The listing builds one solid part. Answer for the finished solid, in the listing's coordinates (mm). Face numbers are marked on the shaded views. Give positions to 0.01 mm unless a question says otherwise; leave off trailing zeros. Loops run counter-clockwise (first coordinate to the right, second up) from the corner with the lowest first, then second, coordinate; pieces in that order, holes last. Notation, with made-up numbers: M 12,-4 L 38,-4 A22 cw 38,15 Z; hole C 13,50 d4. An arc over 180 degrees is marked long. Return JSON: item names as keys, results as strings.
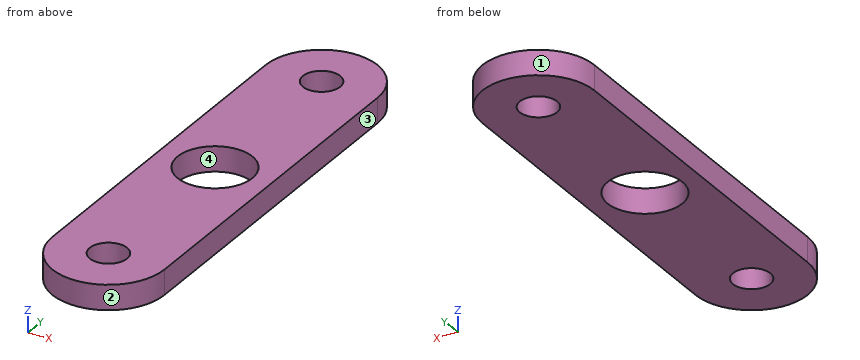
Autodesk Inventor part; units mm, degrees
ref_plane "YZ Plane" through (0, 0, 0) normal (1, 0, 0) x (0, 1, 0)
ref_plane "XZ Plane" through (0, 0, 0) normal (0, 1, 0) x (-1, 0, 0)
ref_plane "XY Plane" through (0, 0, 0) normal (0, 0, 1) x (1, 0, 0)
sketch "Skizze1" plane through (0, 0, 0) normal (0, 0, 1) x (1, 0, 0)
  line L0 (0, -14.25) -> (0, 14.25) construction
  line L1 (4.5, -14.25) -> (4.5, 14.25)
  line L2 (-4.5, 14.25) -> (-4.5, -14.25)
  arc A0 (-4.5, -14.25) -> (4.5, -14.25) centre (0, -14.25) ccw
  arc A1 (4.5, 14.25) -> (-4.5, 14.25) centre (0, 14.25) ccw
  line L3 (0, 28.35) -> (0, -28.35) construction
  line L4 (-8.4, 0) -> (8.4, 0) construction
  circle A2 centre (0, 14.25) radius 1.5
  circle A3 centre (0, -14.25) radius 1.5
  circle A4 centre (0, 0) radius 3
  circle A5 centre (0, 14.25) radius 6 construction
  circle A6 centre (0, -14.25) radius 6 construction
  line L5 (0, 20.25) -> (0, -20.25) construction
  dimension "d4" = 12
  dimension "d1" = 3
  dimension "d2" = 3
  dimension "d3" = 6
  dimension "d5" = 40.5
extrude "Extrusion1" add sketch "Skizze1" along normal blind 2
properties part number "HarmonicDrive-WaveGenerator"
(1) Straight lines are drawn through the part: line 1 along Y through (x, z) = (0, 1.2); line 2 along Y through (x, z) = (-0.75, 1.6); line 3 along X through (y, z) = (1, 0.9). For each, find the intervals that lie inside material, in ascending order.
Values follow:
{"line 1": "-18.75 to -15.75, -12.75 to -3, 3 to 12.75, 15.75 to 18.75", "line 2": "-18.69 to -15.55, -12.95 to -2.9, 2.9 to 12.95, 15.55 to 18.69", "line 3": "-4.5 to -2.83, 2.83 to 4.5"}
(2) The part is cut by section D-D (x = -2). Determine the outline of the cut face in (y, z).
Values follow:
{"outline": "M -18.28,0 L -2.24,0 L -2.24,2 L -18.28,2 Z; M 2.24,0 L 18.28,0 L 18.28,2 L 2.24,2 Z"}
(3) Determine the mould class of the marked faces 1, 2, 3 and 4 for opening direction Y: released by +Y, released by -Y, zero draft, split by the parting line, or undercut.
Values follow:
{"face 1": "released by +Y", "face 2": "released by -Y", "face 3": "zero draft", "face 4": "undercut"}
(4) The part is cut by section B-B (y = 0). Determine the outline of the cut face in (x, z), and give its area (3 significant figures).
Values follow:
{"outline": "M -4.5,0 L -3,0 L -3,2 L -4.5,2 Z; M 3,0 L 4.5,0 L 4.5,2 L 3,2 Z", "area": "6.00 mm²"}
(5) The part is cut by section A-A (x = 0). Determine the outline of the cut face in (y, z), and give its area (3 significant figures).
Values follow:
{"outline": "M -18.75,0 L -15.75,0 L -15.75,2 L -18.75,2 Z; M -12.75,0 L -3,0 L -3,2 L -12.75,2 Z; M 3,0 L 12.75,0 L 12.75,2 L 3,2 Z; M 15.75,0 L 18.75,0 L 18.75,2 L 15.75,2 Z", "area": "51.0 mm²"}
(6) The part is cut by section C-C (z = 0.7). Determine the outline of the cut face in (x, y), and give its area (3 significant figures).
Values follow:
{"outline": "M -4.5,-14.25 A4.5 ccw 4.5,-14.25 L 4.5,14.25 A4.5 ccw -4.5,14.25 Z; hole C 0,0 d6; hole C 0,-14.25 d3; hole C 0,14.25 d3", "area": "278 mm²"}
